The listing builds one solid part. Answer for the finished solid, in the listing's coordinates (mm). Give positions to 0.01 mm unless a question says otherwise; leave off trailing zeros. Loops run counter-clockwise (first coordinate to the right, second up) from the corner with the lowest first, then second, coordinate; pieces in that order, holes last. Notation, with made-up numbers: M 7,13.5 L 24,13.5 A20 ccw 24,30.5 Z; hole C 31,0.5 d2. An arc over 180 degrees is marked long. Return JSON: item names as keys, results as strings.
from build123d import *

# Parameters (mm, degrees)
SKETCH1_W          = 35.56
SKETCH1_H          = 90.932
EXTRUDE1_DEPTH     = 3.175
SKETCH2_W          = 3.175
SKETCH2_H          = 13.208
CUT_EXTRUDE1_DEPTH = 4.175
SKETCH3_W          = 3.175
SKETCH3_H          = 4.885047255
SKETCH3_H_2        = 4.792331668
CUT_EXTRUDE2_DEPTH = 33.385


with BuildPart() as part:
    # Sketch1 → Extrude1 (new body)
    with BuildSketch(Plane(origin=(0, 0, 0), x_dir=(0, 0, -1), z_dir=(1, 0, 0))):
        Rectangle(SKETCH1_W, SKETCH1_H)
    extrude(amount=EXTRUDE1_DEPTH)

    # Sketch2 → Cut-Extrude1 (cut, through all)
    with BuildSketch(Plane(origin=(3.175, 0, 0), x_dir=(0, 0, -1), z_dir=(1, 0, 0))):
        with Locations((-16.1925, 38.862)):
            Rectangle(SKETCH2_W, SKETCH2_H)
        with Locations((-16.1925, 12.954)):
            Rectangle(SKETCH2_W, SKETCH2_H)
        with Locations((-16.1925, -12.954)):
            Rectangle(SKETCH2_W, SKETCH2_H)
        with Locations((-16.1925, -38.862)):
            Rectangle(SKETCH2_W, SKETCH2_H)
        with Locations((-16.1925, -64.77)):
            Rectangle(SKETCH2_W, SKETCH2_H)
        with Locations((16.1925, -38.862)):
            Rectangle(SKETCH2_W, SKETCH2_H)
        with Locations((16.1925, -12.954)):
            Rectangle(SKETCH2_W, SKETCH2_H)
        with Locations((16.1925, 12.954)):
            Rectangle(SKETCH2_W, SKETCH2_H)
        with Locations((16.1925, 38.862)):
            Rectangle(SKETCH2_W, SKETCH2_H)
    extrude(amount=-CUT_EXTRUDE1_DEPTH, mode=Mode.SUBTRACT)

    # Sketch3 → Cut-Extrude2 (cut, through all)
    with BuildSketch(Plane.XY.offset(14.605)):
        with Locations((1.5875, 43.023476372)):
            Rectangle(SKETCH3_W, SKETCH3_H)
        with Locations((1.5875, -43.069834166)):
            Rectangle(SKETCH3_W, SKETCH3_H_2)
    extrude(amount=-CUT_EXTRUDE2_DEPTH, mode=Mode.SUBTRACT)


solid = part.part
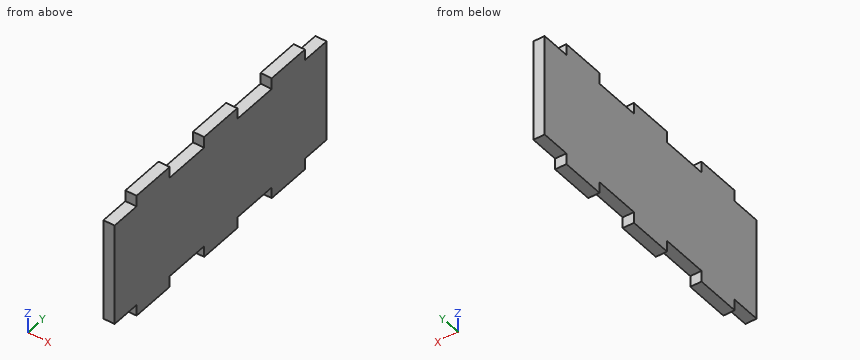
(1) The part is cut by section B-B (y = 17). Determine the outline of the cut face in (x, z) (3 decimals).
Values follow:
{"outline": "M 0,-14.605 L 3.175,-14.605 L 3.175,14.605 L 0,14.605 Z"}
(2) The part is cut by section A-A (x = 1.4). Determine the outline of the cut face in (y, z) (3 decimals), and give its area (3 significant figures).
Values follow:
{"outline": "M -40.674,-14.605 L -32.258,-14.605 L -32.258,-17.78 L -19.558,-17.78 L -19.558,-14.605 L -6.35,-14.605 L -6.35,-17.78 L 6.35,-17.78 L 6.35,-14.605 L 19.558,-14.605 L 19.558,-17.78 L 32.258,-17.78 L 32.258,-14.605 L 40.581,-14.605 L 40.581,14.605 L 32.258,14.605 L 32.258,17.78 L 19.558,17.78 L 19.558,14.605 L 6.35,14.605 L 6.35,17.78 L -6.35,17.78 L -6.35,14.605 L -19.558,14.605 L -19.558,17.78 L -32.258,17.78 L -32.258,14.605 L -40.674,14.605 Z", "area": "2,620 mm²"}
(3) Straight lines are drawn through the part: line 1 along Y through (x, z) = (0.95, 16.5); line 2 along Z through (x, y) = (1.3, 32.5) (3 decimals). For each, find the intervals that lie inside material, in ascending order.
Values follow:
{"line 1": "-32.26 to -19.56, -6.35 to 6.35, 19.56 to 32.26", "line 2": "-14.605 to 14.605"}
(4) Given pin 1 (1.6 mm diameter, centred on x = 2, z = 16.5, fed in from -Y); pin 2 (1.6 mm diameter, centred on x = 1.5, z = 16, fed in from +Y); pin 3 (1 mm diameter, centred on x = 2, y = -9.5, fed in from -Z) (3 decimals), each flat-ended and moving along its own axis, determine where each tip first touches the part or whether it passes through.
Values follow:
{"pin 1": "y = -32.26", "pin 2": "y = 32.26", "pin 3": "z = -14.605"}
